from build123d import *

# Parameters (mm, degrees)
SKETCH_1_W          = 200
SKETCH_1_H          = 250
EXTRUDE_1_DEPTH     = 20
CUT_EXTRUDE_1_REACH = 163.323
SKETCH_2_R          = 7
CHAMFER_1_SIZE      = 5


with BuildPart() as part:
    # 草图1 → 凸台-拉伸1 (new body)
    with BuildSketch(Plane.XY):
        Rectangle(SKETCH_1_W, SKETCH_1_H)
    extrude(amount=EXTRUDE_1_DEPTH)

    # 草图2 → 切除-拉伸1 (cut, up to next)
    with BuildSketch(Plane.XY.offset(20), mode=Mode.PRIVATE) as cut_extrude_1_sk1:
        with Locations((-70, 95)):
            Circle(SKETCH_2_R)
    cut_extrude_1_tool1 = extrude(cut_extrude_1_sk1.sketch, amount=-CUT_EXTRUDE_1_REACH, mode=Mode.PRIVATE) & part.part
    # 草图2 → 切除-拉伸1 (cut, up to next)
    with BuildSketch(Plane.XY.offset(20), mode=Mode.PRIVATE) as cut_extrude_1_sk2:
        with Locations((0, 95)):
            Circle(SKETCH_2_R)
    cut_extrude_1_tool2 = extrude(cut_extrude_1_sk2.sketch, amount=-CUT_EXTRUDE_1_REACH, mode=Mode.PRIVATE) & part.part
    # 草图2 → 切除-拉伸1 (cut, up to next)
    with BuildSketch(Plane.XY.offset(20), mode=Mode.PRIVATE) as cut_extrude_1_sk3:
        with Locations((70, 95)):
            Circle(SKETCH_2_R)
    cut_extrude_1_tool3 = extrude(cut_extrude_1_sk3.sketch, amount=-CUT_EXTRUDE_1_REACH, mode=Mode.PRIVATE) & part.part
    # 草图2 → 切除-拉伸1 (cut, up to next)
    with BuildSketch(Plane.XY.offset(20), mode=Mode.PRIVATE) as cut_extrude_1_sk4:
        with Locations((-70, 35)):
            Circle(SKETCH_2_R)
    cut_extrude_1_tool4 = extrude(cut_extrude_1_sk4.sketch, amount=-CUT_EXTRUDE_1_REACH, mode=Mode.PRIVATE) & part.part
    # 草图2 → 切除-拉伸1 (cut, up to next)
    with BuildSketch(Plane.XY.offset(20), mode=Mode.PRIVATE) as cut_extrude_1_sk5:
        with Locations((70, 35)):
            Circle(SKETCH_2_R)
    cut_extrude_1_tool5 = extrude(cut_extrude_1_sk5.sketch, amount=-CUT_EXTRUDE_1_REACH, mode=Mode.PRIVATE) & part.part
    # 草图2 → 切除-拉伸1 (cut, up to next)
    with BuildSketch(Plane.XY.offset(20), mode=Mode.PRIVATE) as cut_extrude_1_sk6:
        with Locations((-70, -35)):
            Circle(SKETCH_2_R)
    cut_extrude_1_tool6 = extrude(cut_extrude_1_sk6.sketch, amount=-CUT_EXTRUDE_1_REACH, mode=Mode.PRIVATE) & part.part
    # 草图2 → 切除-拉伸1 (cut, up to next)
    with BuildSketch(Plane.XY.offset(20), mode=Mode.PRIVATE) as cut_extrude_1_sk7:
        with Locations((0, -95)):
            Circle(SKETCH_2_R)
    cut_extrude_1_tool7 = extrude(cut_extrude_1_sk7.sketch, amount=-CUT_EXTRUDE_1_REACH, mode=Mode.PRIVATE) & part.part
    # 草图2 → 切除-拉伸1 (cut, up to next)
    with BuildSketch(Plane.XY.offset(20), mode=Mode.PRIVATE) as cut_extrude_1_sk8:
        with Locations((-70, -95)):
            Circle(SKETCH_2_R)
    cut_extrude_1_tool8 = extrude(cut_extrude_1_sk8.sketch, amount=-CUT_EXTRUDE_1_REACH, mode=Mode.PRIVATE) & part.part
    # 草图2 → 切除-拉伸1 (cut, up to next)
    with BuildSketch(Plane.XY.offset(20), mode=Mode.PRIVATE) as cut_extrude_1_sk9:
        with Locations((70, -35)):
            Circle(SKETCH_2_R)
    cut_extrude_1_tool9 = extrude(cut_extrude_1_sk9.sketch, amount=-CUT_EXTRUDE_1_REACH, mode=Mode.PRIVATE) & part.part
    # 草图2 → 切除-拉伸1 (cut, up to next)
    with BuildSketch(Plane.XY.offset(20), mode=Mode.PRIVATE) as cut_extrude_1_sk10:
        with Locations((70, -95)):
            Circle(SKETCH_2_R)
    cut_extrude_1_tool10 = extrude(cut_extrude_1_sk10.sketch, amount=-CUT_EXTRUDE_1_REACH, mode=Mode.PRIVATE) & part.part
    # 草图2 → 切除-拉伸1 (cut, up to next)
    with BuildSketch(Plane.XY.offset(20), mode=Mode.PRIVATE) as cut_extrude_1_sk11:
        with BuildLine():
            Line((-41, 76), (41, 76))
            ThreePointArc((41, 76), (48.071067812, 73.071067812), (51, 66))
            Line((51, 66), (51, -66))
            ThreePointArc((51, -66), (48.071067812, -73.071067812), (41, -76))
            Line((41, -76), (-41, -76))
            ThreePointArc((-41, -76), (-48.071067812, -73.071067812), (-51, -66))
            Line((-51, -66), (-51, 66))
            ThreePointArc((-51, 66), (-48.071067812, 73.071067812), (-41, 76))
        make_face()
    cut_extrude_1_tool11 = extrude(cut_extrude_1_sk11.sketch, amount=-CUT_EXTRUDE_1_REACH, mode=Mode.PRIVATE) & part.part
    add(cut_extrude_1_tool1.solids().sort_by_distance((-70, 95, 20))[0], mode=Mode.SUBTRACT)
    add(cut_extrude_1_tool2.solids().sort_by_distance((0, 95, 20))[0], mode=Mode.SUBTRACT)
    add(cut_extrude_1_tool3.solids().sort_by_distance((70, 95, 20))[0], mode=Mode.SUBTRACT)
    add(cut_extrude_1_tool4.solids().sort_by_distance((-70, 35, 20))[0], mode=Mode.SUBTRACT)
    add(cut_extrude_1_tool5.solids().sort_by_distance((70, 35, 20))[0], mode=Mode.SUBTRACT)
    add(cut_extrude_1_tool6.solids().sort_by_distance((-70, -35, 20))[0], mode=Mode.SUBTRACT)
    add(cut_extrude_1_tool7.solids().sort_by_distance((0, -95, 20))[0], mode=Mode.SUBTRACT)
    add(cut_extrude_1_tool8.solids().sort_by_distance((-70, -95, 20))[0], mode=Mode.SUBTRACT)
    add(cut_extrude_1_tool9.solids().sort_by_distance((70, -35, 20))[0], mode=Mode.SUBTRACT)
    add(cut_extrude_1_tool10.solids().sort_by_distance((70, -95, 20))[0], mode=Mode.SUBTRACT)
    add(cut_extrude_1_tool11.solids().sort_by_distance((0, 0, 20))[0], mode=Mode.SUBTRACT)

    # 倒角1
    chamfer_1_edges = [part.edges().sort_by_distance(p)[0] for p in [
        (0, -125, 20),
        (0, 125, 20),
    ]]
    chamfer(chamfer_1_edges, length=CHAMFER_1_SIZE)


solid = part.part
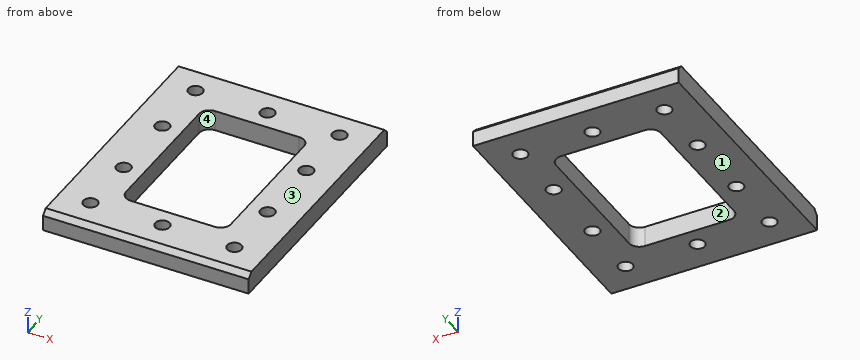
Verification items for the finished model (mm, model axes). Face numbers are marked on the shaded views. A direction names the side the tool comes from. Give positions to 0.01 mm unless a question says otherwise; leave off trailing zeros. Order: outer loops, then holes, each group sorted by start corner. A loop starts at its lowest first (then second) coordinate and runs counter-clockwise, first axis right, second up. Notation, with made-up numbers: M 11,36.5 L 22,36.5 A12 cw 22,57.5 Z; hole C -29,3.25 d4. An arc over 180 degrees is marked long. Answer as a JSON object with one key per item and string values. Group by question number.
1) Access from +Z, -Z, +X, -X, +Y, -Y to the whole of each face (thin tool, end or side, straight path). Record for the marked faces 3 and 4.
2) Mould release check, pull along X, two halves, no side actions. Record for the marked faces 1 and 2: released by +X, released by -X, zero draft, split by the parting line, or undercut.
3) Cross-section at D-D (x = 70). Enter the section's corners in (y, z).
4) Depth check by flat-ended pin: pin 1 Ø11 at (x, y) = (-70, 95) entering from +Z. Enter the tip coordinate at first touch or a pass-through.
5) Cross-section at B-B (x = 0). Enter the section's corners in (y, z), then the cut area to 4 significant figures.
6) Cross-section at A-A (y = 17). Enter the section's corners in (x, z), then the cut area to 3 significant figures.
7) Cross-section at C-C (z = 5.25). Give the number of separate pieces and of enclosed holes in the cut face, then the cut area to 3 significant figures.
8) Scan lines: line 1 along Y through (x, z) = (70, 6.75); line 2 along Y through (x, z) = (-36, 3.75); line 3 along Y through (x, z) = (69, 11). Record each from-to range of solid material in increasing order. Write a range as [from, to].
Result sheet:
{
 "1": {"face 3": "+Z, +X, -X, +Y, -Y", "face 4": "+Z, -Z"},
 "2": {"face 1": "zero draft", "face 2": "undercut"},
 "3": {"outline": "M -125,0 L -102,0 L -102,20 L -120,20 L -125,15 Z; M -88,0 L -42,0 L -42,20 L -88,20 Z; M -28,0 L 28,0 L 28,20 L -28,20 Z; M 42,0 L 88,0 L 88,20 L 42,20 Z; M 102,0 L 125,0 L 125,15 L 120,20 L 102,20 Z"},
 "4": {"pin 1": "passes through"},
 "5": {"outline": "M -125,0 L -102,0 L -102,20 L -120,20 L -125,15 Z; M -88,0 L -76,0 L -76,20 L -88,20 Z; M 76,0 L 88,0 L 88,20 L 76,20 Z; M 102,0 L 125,0 L 125,15 L 120,20 L 102,20 Z", "area": "1,375 mm2"},
 "6": {"outline": "M -100,0 L -51,0 L -51,20 L -100,20 Z; M 51,0 L 100,0 L 100,20 L 51,20 Z", "area": "1,960 mm2"},
 "7": {"separate pieces": "1", "enclosed holes": "11", "area": "33,000 mm2"},
 "8": {"line 1": "y = [-125, -102], [-88, -42], [-28, 28], [42, 88], [102, 125]", "line 2": "y = [-125, -76], [76, 125]", "line 3": "y = [-125, -101.93], [-88.07, -41.93], [-28.07, 28.07], [41.93, 88.07], [101.93, 125]"}
}
